Geometry: final body of the model. Coordinates: model frame, mm. Face numbers are marked on the shaded views. A direction names the side the tool comes from. Round coordinates to 2 decimals unless told otherwise and drop trailing zeros. Loops run counter-clockwise (first coordinate to the right, second up) from the corner with the lowest first, then second, coordinate; pieces in that order, holes last. Notation, with made-up numbers: M -19.5,32 L 10.5,32 A21 ccw 10.5,60 Z; hole C 49,-12 d6. An arc over 180 degrees is marked long. Return JSON: item names as keys, results as strings.
from build123d import *

# Parameters (mm, degrees)
F0_W      = 203.2
F0_H      = 25.4
F1_DEPTH  = 81.28
F3_DEPTH  = 203.2
F5_DEPTH  = 83.82
F6_DEPTH  = 78.74
F7_DEPTH  = 2.54
F8_DEPTH  = 2.54
F9_DEPTH  = 60.96
F11_DEPTH = 60.96


with BuildPart() as f1:
    # F0 (on Front) → F1 (new body)
    with BuildSketch(Plane.XZ):
        with Locations((-14.4892223179, -13.8418302595)):
            Rectangle(F0_W, F0_H)
    extrude(amount=-F1_DEPTH)

    # F2 (on face) → F3 (join)
    with BuildSketch(Plane.YZ.offset(87.1107776821)):
        Polygon((0, -1.1418302595), (81.28, -1.1418302595), (40.64, 25.5536600589), align=None)
    extrude(amount=-F3_DEPTH)

    # F4 (on face) → F5 (join)
    with BuildSketch(Plane.XZ):
        Polygon((13.4507776821, 25.6081018597), (-24.6492223179, -1.1418302595), (-20.2288646721, -1.1418302595), (13.4507776821, 22.5045777922), (47.1304200362, -1.1418302595), (51.5507776821, -1.1418302595), align=None)
    extrude(amount=-F5_DEPTH)

    # F4 (on face) → F6 (join)
    with BuildSketch(Plane.XZ):
        Polygon((13.4507776821, 22.5045777922), (-20.2288646721, -1.1418302595), (47.1304200362, -1.1418302595), align=None)
    extrude(amount=-F6_DEPTH)

    # F4 (on face) → F7 (cut)
    with BuildSketch(Plane.XZ):
        Polygon((13.4507776821, 22.5045777922), (-20.2288646721, -1.1418302595), (47.1304200362, -1.1418302595), align=None)
    extrude(amount=-F7_DEPTH, mode=Mode.SUBTRACT)

    # F4 (on face) → F8 (join)
    with BuildSketch(Plane.XZ):
        Polygon((13.4507776821, 25.6081018597), (-24.6492223179, -1.1418302595), (-20.2288646721, -1.1418302595), (13.4507776821, 22.5045777922), (47.1304200362, -1.1418302595), (51.5507776821, -1.1418302595), align=None)
    extrude(amount=F8_DEPTH)

    # F9 (cut): a face of the model
    f9_faces = [f1.faces().sort_by_distance(p)[0] for p in [
        (-116.0892223179, 40.64, -6.4016236214),
    ]]
    extrude(f9_faces, amount=-F9_DEPTH, mode=Mode.SUBTRACT)

    # F10 (on face) → F11 (join)
    with BuildSketch(Plane(origin=(-55.1292223179, 0, 0), x_dir=(0, -1, 0), z_dir=(-1, 0, 0))):
        Polygon((-40.64, 19.6767237691), (-76.2, -3.6818302595), (-76.2, -26.5418302595), (-5.08, -26.5418302595), (-5.08, -3.6818302595), align=None)
    extrude(amount=F11_DEPTH)


solid = f1.part
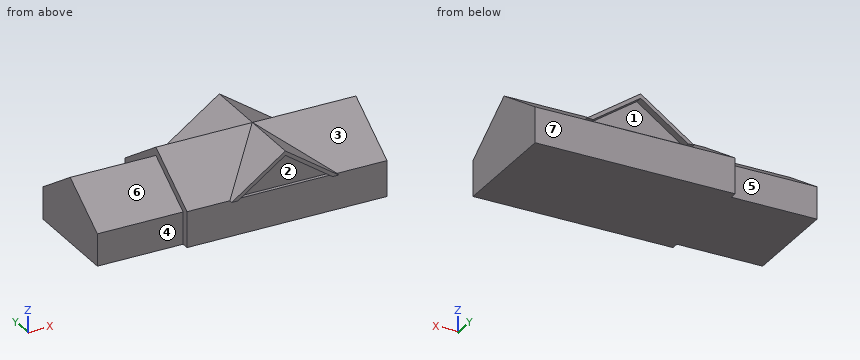
Q1. Section query A-A (z = -18). Output: boundary loops of the cut face in (x, y), plus the area to 3 significant figures.
Determined:
{"outline": "M -116.09,5.08 L -55.13,5.08 L -55.13,0 L 87.11,0 L 87.11,81.28 L -55.13,81.28 L -55.13,76.2 L -116.09,76.2 Z", "area": "15,900 mm^2"}
Q2. Section query B-B (x = -39.5). Output: boundary loops of the cut face in (y, z).
Determined:
{"outline": "M 0,-26.54 L 81.28,-26.54 L 81.28,-1.14 L 40.64,25.55 L 0,-1.14 Z"}
Q3. Section query C-C (y = 43). Output: boundary loops of the cut face in (x, z), plus the area to 3 significant figures.
Determined:
{"outline": "M -116.09,-26.54 L 87.11,-26.54 L 87.11,24 L 15.74,24 L 13.45,25.61 L 11.17,24 L -55.13,24 L -55.13,18.13 L -116.09,18.13 Z", "area": "9,920 mm^2"}
Q4. Material intervals for L1, parallel to Y at x = -89, z = -12; L2, parallel to Y at x = 65.5, z = -1.5; L3, parallel to X at y = 80, z = -9, sorted ascending.
Determined:
{"L1": "y = 5.08 to 76.2", "L2": "y = 0 to 81.28", "L3": "x = -55.13 to 87.11"}
Q5. Reachability of the marked faces 5, 6 and 7 from +Z, -Z, +X, -X, +Y, -Y: full face, straight path, thin tool, end or side. Return the list, or none.
Determined:
{"face 5": "+Z, -Z, -X, +Y", "face 6": "+Z, -X, -Y", "face 7": "-Z, +X, -X, +Y"}
Q6. Pull-direction query (Z, two-part tool) for the marked faces 1, 2, 3 and 4; classes: pulls with the +Z half, pulls with the -Z half, needs draft (parallel to the pull), parting line crosses it, or undercut.
Determined:
{"face 1": "undercut", "face 2": "undercut", "face 3": "pulls with the +Z half", "face 4": "needs draft"}
Q7. Pin query (flat end, axial travel): pin 1 (25 mm diameter, centred on x = -80, z = -16, fed in from -Y); pin 2 (1.3 mm diameter, centred on x = 49, y = 82.5, fed in from -Z); pin 3 (3 mm diameter, centred on x = 28.5, y = 1.5, fed in from +Z). Return the tip coordinate at first contact, or that it passes through.
Determined:
{"pin 1": "stops at y = 5.08", "pin 2": "stops at z = -1.14", "pin 3": "stops at z = 16.1"}
Q8. Section query D-D (x = -101). Output: boundary loops of the cut face in (y, z), plus the area to 3 significant figures.
Determined:
{"outline": "M 5.08,-26.54 L 76.2,-26.54 L 76.2,-3.68 L 40.64,19.68 L 5.08,-3.68 Z", "area": "2,460 mm^2"}
